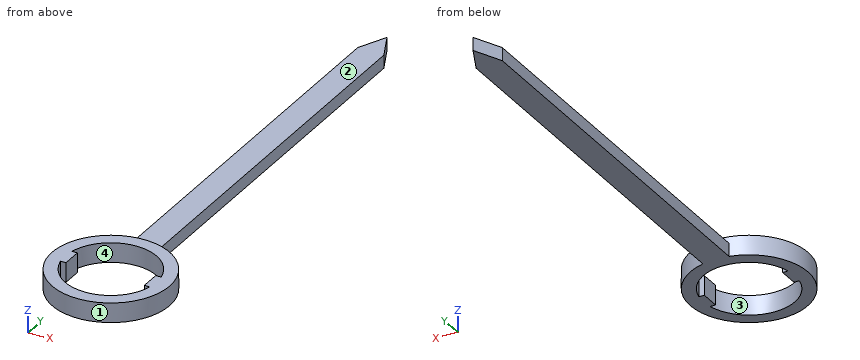
from build123d import *

# Parameters (mm, degrees)
SKETCH1_R           = 9
BOSS_EXTRUDE1_DEPTH = 3
BOSS_EXTRUDE2_DEPTH = 2


with BuildPart() as part:
    # Sketch1 → Boss-Extrude1 (new body)
    with BuildSketch(Plane.XY):
        Circle(SKETCH1_R)
        with BuildLine():
            Line((-6.837397166, -1.5), (-8, -1.5))
            Line((-8, -1.5), (-8, 1.5))
            Line((-8, 1.5), (-6.837397166, 1.5))
            ThreePointArc((-6.837397166, 1.5), (0, 7), (6.837397166, 1.5))
            Line((6.837397166, 1.5), (8, 1.5))
            Line((8, 1.5), (8, -1.5))
            Line((8, -1.5), (6.837397166, -1.5))
            ThreePointArc((6.837397166, -1.5), (0, -7), (-6.837397166, -1.5))
        make_face(mode=Mode.SUBTRACT)
        with BuildLine():
            Line((6, -1.5), (6.837397166, -1.5))
            ThreePointArc((6.837397166, -1.5), (6.959230567, -0.754393744), (7, 0))
            ThreePointArc((7, 0), (6.959230567, 0.754393744), (6.837397166, 1.5))
            Line((6.837397166, 1.5), (6, 1.5))
            Line((6, 1.5), (6, -1.5))
        make_face()
        with BuildLine():
            ThreePointArc((7, 0), (6.959230567, -0.754393744), (6.837397166, -1.5))
            Line((6.837397166, -1.5), (8, -1.5))
            Line((8, -1.5), (8, 1.5))
            Line((8, 1.5), (6.837397166, 1.5))
            ThreePointArc((6.837397166, 1.5), (6.959230567, 0.754393744), (7, 0))
        make_face()
        with BuildLine():
            Line((-8, 1.5), (-8, -1.5))
            Line((-8, -1.5), (-6.837397166, -1.5))
            ThreePointArc((-6.837397166, -1.5), (-7, 0), (-6.837397166, 1.5))
            Line((-6.837397166, 1.5), (-8, 1.5))
        make_face()
        with BuildLine():
            ThreePointArc((-6.837397166, 1.5), (-7, 0), (-6.837397166, -1.5))
            Line((-6.837397166, -1.5), (-6, -1.5))
            Line((-6, -1.5), (-6, 1.5))
            Line((-6, 1.5), (-6.837397166, 1.5))
        make_face()
    extrude(amount=BOSS_EXTRUDE1_DEPTH)

    # Sketch2 → Boss-Extrude2 (add)
    with BuildSketch(Plane(origin=(0, 0, 0), x_dir=(-1, 0, 0), z_dir=(0, 0, -1))):
        with BuildLine():
            Line((-2, 68.774964387), (-2, 8.774964387))
            ThreePointArc((-2, 8.774964387), (0, 9), (2, 8.774964387))
            Line((2, 8.774964387), (2, 68.774964387))
            Line((2, 68.774964387), (0, 73.063978228))
            Line((0, 73.063978228), (-2, 68.774964387))
        make_face()
    extrude(amount=-BOSS_EXTRUDE2_DEPTH)


solid = part.part
The model under review builds one solid part; all positions refer to its coordinate system, in mm. Face numbers are marked on the shaded views. Give positions to 0.01 mm unless a question says otherwise; leave off trailing zeros. Write each loop counter-clockwise with the first axis right and the second up, starting at its lowest first coordinate (ties: lowest second). Pieces come first, ordered by that corner, then holes.
1. Add section A-A, the plane y = 0. Write out the cut boundary in (x, z).
2. Add section D-D, the plane x = -3.75. Write out the cut boundary in (y, z).
3. For P1, Ø3, axis at x = -1, y = 38, coming from the +Z side; P2, Ø4, axis at x = -5, y = 48.5, coming from the -Z side; P3, Ø0.9, axis at x = -6.5, z = 1, coming from the -Y side; P4, Ø0.7, axis at x = 6.5, z = 2, coming from the -Y side, all flat-tipped, find the tip position at first contact; note any pin that passes through.
4. Wall thickness on L1, parallel to X at y = 68, z = 1.25; L2, parallel to Y at x = 5.25, z = 0.45; L3, parallel to Y at x = 2.5, z = 0.55: over which ranges is each line inside the solid? List them lowest first.
5. Draft analysis for pull direction Y (two halves, no side actions). For the marked faces 1, 2, 3 and 4, state which applies: +Y half, -Y half, draft (parallel to the pull), parting line (faces both ways), or undercut.
6. Add section B-B, the plane z = 0.65. Write out the cut boundary in (x, y), plus the area to 3 significant figures.
7. Add section C-C, the plane x = -0.75. Write out the cut boundary in (y, z).
Worked answers:
1. outline: (-9, 0) - (-6, 0) - (-6, 3) - (-9, 3) - close; (6, 0) - (9, 0) - (9, 3) - (6, 3) - close
2. outline: (-8.18, 0) - (-5.91, 0) - (-5.91, 3) - (-8.18, 3) - close; (5.91, 0) - (8.18, 0) - (8.18, 3) - (5.91, 3) - close
3. P1: stops at z = 2
3. P2: passes through
3. P3: stops at y = -6.66
3. P4: stops at y = -6.57
4. L1: x = -2 to 2
4. L2: y = -7.31 to -4.63, 4.63 to 7.31
4. L3: y = -8.65 to -6.54, 6.54 to 8.65
5. face 1: parting line
5. face 2: draft
5. face 3: undercut
5. face 4: undercut
6. outline: (-2, 8.77) arc R9 ccw (long way) to (2, 8.77) - (2, 68.77) - (0, 73.06) - (-2, 68.77) - close; hole (-6.84, -1.5) arc R7 ccw to (6.84, -1.5) - (6, -1.5) - (6, 1.5) - (6.84, 1.5) arc R7 ccw to (-6.84, 1.5) - (-6, 1.5) - (-6, -1.5) - close
6. area: 354 mm2
7. outline: (-8.97, 0) - (-6.96, 0) - (-6.96, 3) - (-8.97, 3) - close; (6.96, 0) - (71.46, 0) - (71.46, 2) - (8.97, 2) - (8.97, 3) - (6.96, 3) - close
